Build history of the part. All positions in model axes, mm. Face numbers are marked on the shaded views. A direction names the side the tool comes from. Round coordinates to 2 decimals unless told otherwise and drop trailing zeros. Order: outer loops, then holes, each group sorted by start corner. A loop starts at its lowest first (then second) coordinate and runs counter-clockwise, first axis right, second up. Notation, with made-up numbers: (2.5, 78.5) -> (32.5, 78.5) arc R29 cw to (32.5, 110.5) -> close; hole circle Ø11 at (-13.75, 76.25). An arc over 180 degrees is marked (long way). Write item = value, one per line.
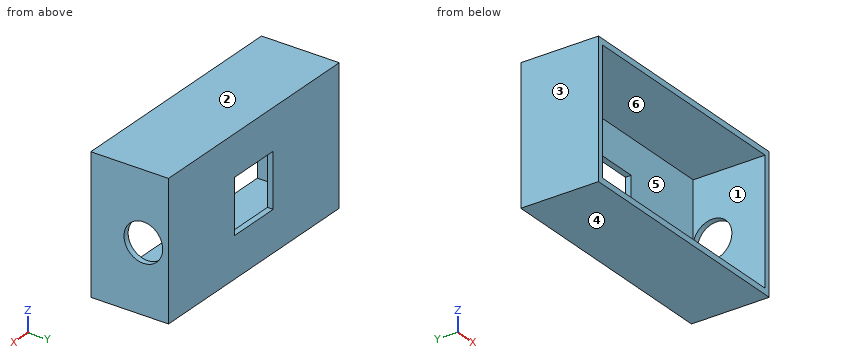
from build123d import *

# Parameters (mm, degrees)
SKETCH_1_W          = 62
SKETCH_1_H          = 35
EXTRUDE_1_DEPTH     = 1.5
SKETCH_2_W          = 62
SKETCH_2_H          = 35
EXTRUDE_2_DEPTH     = 16.1
SKETCH_3_W          = 59
SKETCH_3_H          = 32
CUT_EXTRUDE_1_DEPTH = 41
SKETCH_4_W          = 62
SKETCH_4_H          = 35
SKETCH_4_W_2        = 59
SKETCH_4_H_2        = 32
EXTRUDE_3_DEPTH     = 1
SKETCH_5_W          = 62
SKETCH_5_H          = 35
EXTRUDE_4_DEPTH     = 1.5
SKETCH_8_R          = 5
CUT_EXTRUDE_3_DEPTH = 1.5
CUT_EXTRUDE_4_REACH = 22.1
SKETCH_10_W         = 14
SKETCH_10_H         = 14


with BuildPart() as part:
    # 草图1 → 凸台-拉伸1 (new body)
    with BuildSketch(Plane(origin=(0, 0, 0), x_dir=(1, 0, 0), z_dir=(0, 1, 0))):
        with Locations((2.996831225, 4.751847291)):
            Rectangle(SKETCH_1_W, SKETCH_1_H)
    extrude(amount=EXTRUDE_1_DEPTH)

    # 草图2 → 凸台-拉伸2 (add)
    with BuildSketch(Plane.XZ):
        with Locations((2.996831225, -4.751847291)):
            Rectangle(SKETCH_2_W, SKETCH_2_H)
    extrude(amount=EXTRUDE_2_DEPTH)

    # 草图3 → 切除-拉伸1 (cut)
    with BuildSketch(Plane.XZ.offset(16.1)):
        with Locations((2.996831225, -4.751847291)):
            Rectangle(SKETCH_3_W, SKETCH_3_H)
    extrude(amount=-CUT_EXTRUDE_1_DEPTH, mode=Mode.SUBTRACT)

    # 草图4 → 凸台-拉伸3 (add)
    with BuildSketch(Plane(origin=(0, 1.5, 0), x_dir=(1, 0, 0), z_dir=(0, 1, 0))):
        with Locations((2.996831225, 4.751847291)):
            Rectangle(SKETCH_4_W, SKETCH_4_H)
        with Locations((2.996831225, 4.751847291)):
            Rectangle(SKETCH_4_W_2, SKETCH_4_H_2, mode=Mode.SUBTRACT)
    extrude(amount=EXTRUDE_3_DEPTH)

    # 草图5 → 凸台-拉伸4 (add)
    with BuildSketch(Plane(origin=(0, 2.5, 0), x_dir=(1, 0, 0), z_dir=(0, 1, 0))):
        with Locations((2.996831225, 4.751847291)):
            Rectangle(SKETCH_5_W, SKETCH_5_H)
    extrude(amount=EXTRUDE_4_DEPTH)

    # 草图8 → 切除-拉伸3 (cut)
    with BuildSketch(Plane(origin=(33.996831225, 0, 0), x_dir=(0, 0, -1), z_dir=(1, 0, 0))):
        with Locations((4.751847291, -2.5)):
            Circle(SKETCH_8_R)
    extrude(amount=-CUT_EXTRUDE_3_DEPTH, mode=Mode.SUBTRACT)

    # 草图10 → 切除-拉伸4 (cut, up to next)
    with BuildSketch(Plane(origin=(0, 4, 0), x_dir=(1, 0, 0), z_dir=(0, 1, 0)), mode=Mode.PRIVATE) as cut_extrude_4_sk1:
        with Locations((2.996831225, 4.751847291)):
            Rectangle(SKETCH_10_W, SKETCH_10_H)
    cut_extrude_4_tool1 = extrude(cut_extrude_4_sk1.sketch, amount=-CUT_EXTRUDE_4_REACH, mode=Mode.PRIVATE) & part.part
    add(cut_extrude_4_tool1.solids().sort_by_distance((2.996831, 4, -4.751847))[0], mode=Mode.SUBTRACT)


solid = part.part
Q1. Cut at B-B, the plane y = -13.5. List the corners of the cut face in (x, z), and give its area (3 significant figures).
Check values:
outline = (-28, -22.25) -> (34, -22.25) -> (34, 12.75) -> (-28, 12.75) -> close; hole (-26.5, -20.75) -> (32.5, -20.75) -> (32.5, 11.25) -> (-26.5, 11.25) -> close
area = 282 mm²
Q2. Cut at D-D, the plane y = -2.5. List the corners of the cut face in (x, z).
Check values:
outline = (-28, -22.25) -> (34, -22.25) -> (34, -9.75) -> (32.5, -9.75) -> (32.5, -20.75) -> (-26.5, -20.75) -> (-26.5, 11.25) -> (32.5, 11.25) -> (32.5, 0.25) -> (34, 0.25) -> (34, 12.75) -> (-28, 12.75) -> close
Q3. Cut at C-C, the plane z = -17.5. List the corners of the cut face in (x, y).
Check values:
outline = (-28, -16.1) -> (-26.5, -16.1) -> (-26.5, 2.5) -> (32.5, 2.5) -> (32.5, -16.1) -> (34, -16.1) -> (34, 4) -> (-28, 4) -> close
Q4. Flat gauge pins, fed straight in: pin 1 (12 mm diameter, centred on x = 25.5, z = 4, fed in from -Y); pin 2 (8 mm diameter, centred on y = -2.5, z = -4.75, fed in from +X). Where does each tip first touch, or does it go through?
Check values:
pin_1 = 2.5
pin_2 = -26.5
Q5. Mould opens along Z. For the marked faces 3, 4, 5 and 6 say: released by +Z, released by -Z, zero draft, split by the parting line, or undercut.
Check values:
face_3 = zero draft
face_4 = released by -Z
face_5 = undercut
face_6 = undercut
Q6. Probe probe 1 along Z at (x, y) = (11, -12.75); probe 2 along X at (y, z) = (-4, 7); probe 3 along Z at (x, y) = (33.7, -2.5). List the from-to ranges inside material, lowest first.
Check values:
probe_1 = -22.25 to -20.75, 11.25 to 12.75
probe_2 = -28 to -26.5, 32.5 to 34
probe_3 = -22.25 to -9.75, 0.25 to 12.75
Q7. Which spindle directions (+Z, -Z, +X, -X, +Y, -Y) get a long thin tool onto all of the face, cutting with end or side? Do the marked faces 1 and 2. Say none if no direction does.
Check values:
face_1 = -Y
face_2 = +Z, +X, -X, +Y, -Y
Q8. Cut at A-A, the plane x = 7.5. List the corners of the cut face in (y, z), and give its area (3 significant figures).
Check values:
outline = (-16.1, -22.25) -> (4, -22.25) -> (4, -11.75) -> (2.5, -11.75) -> (2.5, -20.75) -> (-16.1, -20.75) -> close; (-16.1, 11.25) -> (2.5, 11.25) -> (2.5, 2.25) -> (4, 2.25) -> (4, 12.75) -> (-16.1, 12.75) -> close
area = 87.3 mm²
